Model file for the job. Use its own axes, mm. Coordinates: 2 decimals unless noted, no trailing zeros. Order: outer loops, then holes, each group sorted by start corner. A loop starts at its lowest first (then second) coordinate and runs counter-clockwise, first axis right, second up.
from build123d import *

# Parameters (mm, degrees)
F0_W     = 12.8
F0_H     = 19.5
F0_W_2   = 31
F0_H_2   = 27
F1_DEPTH = 1.5
F2_R     = 1


with BuildPart() as f1:
    # F0 (on Top) → F1 (new body)
    with BuildSketch(Plane.XY):
        with BuildLine():
            Line((-24, -26), (24, -26))
            ThreePointArc((24, -26), (27.535534, -24.535534), (29, -21))
            Line((29, -21), (29, 21))
            ThreePointArc((29, 21), (27.535534, 24.535534), (24, 26))
            Line((24, 26), (-24, 26))
            ThreePointArc((-24, 26), (-27.535534, 24.535534), (-29, 21))
            Line((-29, 21), (-29, -21))
            ThreePointArc((-29, -21), (-27.535534, -24.535534), (-24, -26))
        make_face()
        with Locations((-17, 0)):
            Rectangle(F0_W, F0_H, mode=Mode.SUBTRACT)
        with Locations((7.9, 0)):
            Rectangle(F0_W_2, F0_H_2, mode=Mode.SUBTRACT)
    extrude(amount=F1_DEPTH)

    # F2
    f2_edges = [f1.edges().sort_by_distance(p)[0] for p in [
        (-29, 0, 1.5),
    ]]
    fillet(f2_edges, radius=F2_R)


solid = f1.part
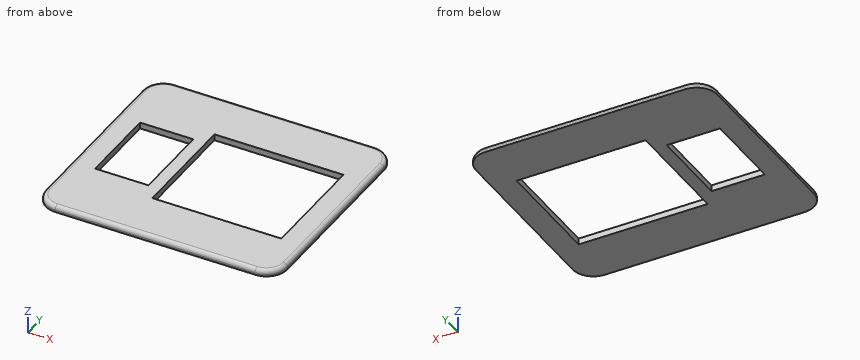
Q1. Cut at C-C, the plane z = 0.85. List the corners of the cut face in (x, y), plus the area to 3 significant figures.
Established:
outline: (-28.94, -21) arc R4.94 ccw to (-24, -25.94) - (24, -25.94) arc R4.94 ccw to (28.94, -21) - (28.94, 21) arc R4.94 ccw to (24, 25.94) - (-24, 25.94) arc R4.94 ccw to (-28.94, 21) - close; hole (-23.4, -9.75) - (-10.6, -9.75) - (-10.6, 9.75) - (-23.4, 9.75) - close; hole (-7.6, -13.5) - (23.4, -13.5) - (23.4, 13.5) - (-7.6, 13.5) - close
area: 1,890 mm2
Q2. Cut at B-B, the plane y = 11.5. List the corners of the cut face in (x, z).
Established:
outline: (-29, 0) - (-7.6, 0) - (-7.6, 1.5) - (-28, 1.5) arc R1 ccw to (-29, 0.5) - close; (23.4, 0) - (29, 0) - (29, 0.5) arc R1 ccw to (28, 1.5) - (23.4, 1.5) - close
Q3. Drop a flat-ended pin along its axis: P1, Ø0.8, axis at y = 5, z = 1, coming from the +X side (3 decimals). Give the stop position or say it passes through.
Established:
P1: stops at x = 28.995
Q4. Probe line 1 (X direction, y = 5, z = 0.6); line 2 (Y direction, x = 7.5, z = 0.1); line 3 (X direction, y = 4, z = 1.1). List the from-to ranges inside material, lowest first.
Established:
line 1: x = -28.99 to -23.4, -10.6 to -7.6, 23.4 to 28.99
line 2: y = -26 to -13.5, 13.5 to 26
line 3: x = -28.8 to -23.4, -10.6 to -7.6, 23.4 to 28.8
Q5. Cut at A-A, the plane x = 14. List the corners of the cut face in (y, z), plus the area to 3 significant figures.
Established:
outline: (-26, 0) - (-13.5, 0) - (-13.5, 1.5) - (-25, 1.5) arc R1 ccw to (-26, 0.5) - close; (13.5, 0) - (26, 0) - (26, 0.5) arc R1 ccw to (25, 1.5) - (13.5, 1.5) - close
area: 37.1 mm2
